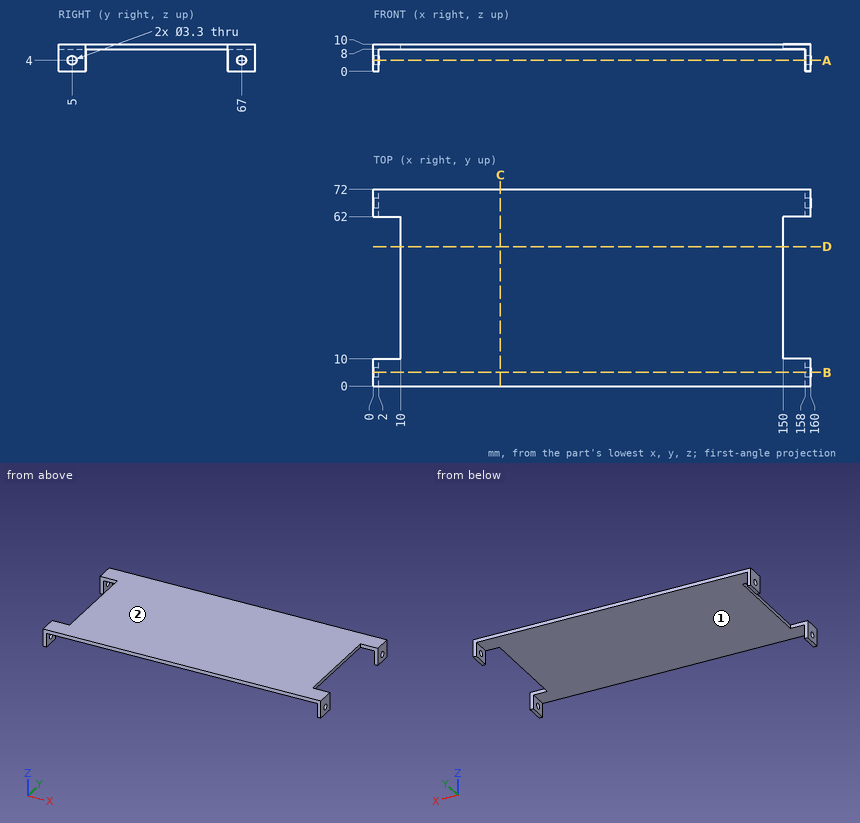
For this review, use the dimensioned drawing (mm, ordinates from the lowest corner) and the shaded views. A direction names the side the tool comes from. Give positions to 0.01 mm unless a question says otherwise; leave off trailing zeros. Order: outer loops, then holes, each group sorted by start corner. A loop starts at its lowest first (then second) coordinate and runs counter-clockwise, first axis right, second up.
1) Take a section at A-A (z = 4). State how many separate pieces and enclosed holes the cut face has, then the cut area to 3 significant figures.
2) Insertion check: pin 1 (2 mm diameter, centred on y = 67, z = 4, fed in from +X); pin 2 (1.6 mm diameter, centred on y = 44.5, z = 8.5, fed in from +X); pin 3 (6 mm diameter, centred on x = 121, y = 47.5, fed in from -Z); pin 4 (2 mm diameter, centred on y = 32.5, z = 9, fed in from -X). Each pin has a flat end and moves straight along its axis. Give the tip position at first contact, or say it passes through.
3) Take a section at B-B (y = 5). Give the boundary of the cut face in (x, z), then the cut area to 3 significant figures.
4) For the marked faces 1 and 2, list the 3-axis set-ups (+Z, -Z, +X, -X, +Y, -Y) from which the entire face can be reached by the end or side of a thin tool; tool diameter is ignored.
5) Wall thickness on line 1 (Z direction, x = 159.6, y = 5); line 2 (Z direction, x = 101, y = 53.5); line 3 (X direction, y = 62.5, z = 7.5): over which ranges is each line inside the solid? List them lowest first.
6) Take a section at C-C (x = 46.5). Give the boundary of the cut face in (y, z).
7) Take a section at D-D (y = 51). Give the boundary of the cut face in (x, z), then the cut area to 3 significant figures.
Derived:
1. separate pieces: 8
1. enclosed holes: 0
1. area: 53.6 mm2
2. pin 1: passes through
2. pin 2: stops at x = 150
2. pin 3: stops at z = 8
2. pin 4: stops at x = 10
3. outline: (0, 0) - (2, 0) - (2, 2.35) - (0, 2.35) - close; (0, 5.65) - (2, 5.65) - (2, 8) - (158, 8) - (158, 5.65) - (160, 5.65) - (160, 10) - (0, 10) - close; (158, 0) - (160, 0) - (160, 2.35) - (158, 2.35) - close
3. area: 339 mm2
4. face 1: -Z, +Y, -Y
4. face 2: +Z, +X, -X, +Y, -Y
5. line 1: z = 0 to 2.35, 5.65 to 10
5. line 2: z = 8 to 10
5. line 3: x = 0 to 2, 158 to 160
6. outline: (0, 8) - (72, 8) - (72, 10) - (0, 10) - close
7. outline: (10, 8) - (150, 8) - (150, 10) - (10, 10) - close
7. area: 280 mm2
